Part model, mm, in its own coordinate system. A direction names the side the tool comes from. Coordinates: 2 decimals unless noted, no trailing zeros. Order: outer loops, then holes, each group sorted by start corner. A loop starts at its lowest first (then second) coordinate and runs counter-clockwise, first axis right, second up. Notation, with made-up numbers: M 7,83 L 61,83 A19 cw 61,115 Z; hole C 59.5,-37 d5. An arc over 180 degrees is marked long. Answer in a Markdown table with one row per item. Add a question column.
from build123d import *
from OCP.BRepFilletAPI import BRepFilletAPI_MakeChamfer

# Parameters (mm, degrees)
CROQUIS1_R              = 5.48
CROQUIS1_R_2            = 2.425
SALIENTE_EXTRUIR1_DEPTH = 2.5
CHAFL_N1_SIZE           = 0.4
CHAFL_N1_SIZE2          = 0.692820323
CROQUIS2_R              = 4.265221528
CROQUIS2_R_2            = 3.76303741
SALIENTE_EXTRUIR2_DEPTH = 2.55


with BuildPart() as part:
    # Croquis1 → Saliente-Extruir1 (new, symmetric)
    with BuildSketch(Plane.XY):
        Circle(CROQUIS1_R)
        Circle(CROQUIS1_R_2, mode=Mode.SUBTRACT)
    extrude(amount=SALIENTE_EXTRUIR1_DEPTH, both=True)

    # Chaflán1: one chamfer whose edges measure the first distance from different faces: ONE call of the kernel's chamfer builder (chamfer() names one face for all edges)
    chafl_n1_edges_1 = [part.edges().sort_by_distance(p)[0] for p in [
        (-5.48, 0, -2.5),
    ]]
    chafl_n1_side_1 = [part.faces().sort_by_distance(p)[0] for p in [
        (-5.325002194, 0, -2.5),
    ]]
    chafl_n1_edges_2 = [part.edges().sort_by_distance(p)[0] for p in [
        (-5.48, 0, 2.5),
    ]]
    chafl_n1_side_2 = [part.faces().sort_by_distance(p)[0] for p in [
        (-5.48, 0, 0),
    ]]
    chafl_n1 = BRepFilletAPI_MakeChamfer(part.part.solid().wrapped)
    for e in chafl_n1_edges_1:
        chafl_n1.Add(CHAFL_N1_SIZE, CHAFL_N1_SIZE2, e.wrapped, chafl_n1_side_1[0].wrapped)  # the first distance lies on this face
    for e in chafl_n1_edges_2:
        chafl_n1.Add(CHAFL_N1_SIZE, CHAFL_N1_SIZE2, e.wrapped, chafl_n1_side_2[0].wrapped)  # the first distance lies on this face
    add(Compound.cast(chafl_n1.Shape()), mode=Mode.REPLACE)

    # Croquis2 → Saliente-Extruir2 (add, symmetric)
    with BuildSketch(Plane(origin=(0, 0, 0), x_dir=(-1, 0, 0), z_dir=(0, 0, -1))):
        with Locations(Location((0, 0, 0), (0, 0, 180))):
            Circle(CROQUIS2_R)
        with Locations(Location((0, 0, 0), (0, 0, 180))):
            Circle(CROQUIS2_R_2, mode=Mode.SUBTRACT)
    extrude(amount=SALIENTE_EXTRUIR2_DEPTH, both=True)


solid = part.part
(1) Wall check: line 1 (Y direction, x = 0, z = 0.5) (3 decimals); line 2 (Z direction, x = 1.75, y = -3); line 3 (X direction, y = 0.5, z = -2.2). Give the ranges that are in metal, low to high.
(2) Slice it at C-C (z = 1.1). List the corners of the cut face in (x, y) (3 decimals).
(3) Drop flat-ended pins along their axis: P1, Ø1.5, axis at x = -3, z = 0, coming from the -Y side; P2, Ø3, axis at x = 0, y = 0, coming from the -Z side; P3, Ø6, axis at x = 0, y = 0, coming from the -Z side; P4, Ø3, axis at x = 0, y = -1, coming from the +Z side. Give the stop position or say it passes through.
(4) Pull direction X, two halves, no side cores. Call faces 3 (the flat face through (-4, -2, 2.5)), 4 (the flat face through (0.8, -2.5, -2.5)), 5 (the cylindrical face through (5.227, 1.646, 0.174)): pulls with the +X half, pulls with the -X half, needs draft (parallel to the pull), parting line crosses it, or undercut.
(5) 3-axis set-ups, long thin cutter, end or side, ignore diameter. For faces 1 (the flat face through (0, 4, -2.55)), 2 (the flat face through (0.8, -2.5, 2.5)): which of +Z, -Z, +X, -X, +Y, -Y reach the whole face in a straight line?
(6) Slice it at A-A (x = 0). List the corners of the cut face in (y, z) (3 decimals).
Computed:
| question | item | result |
|---|---|---|
| 1 | line 1 | y = -5.48 to -2.425, 2.425 to 5.48 |
| 1 | line 2 | z = -2.5 to 2.5 |
| 1 | line 3 | x = -5.23 to -2.37, 2.37 to 5.23 |
| 2 | outline | C 0,0 d10.96; hole C 0,0 d4.85 |
| 3 | P1 | stops at y = -5 |
| 3 | P2 | passes through |
| 3 | P3 | stops at z = -2.5 |
| 3 | P4 | stops at z = 2.5 |
| 4 | face 3 | needs draft |
| 4 | face 4 | undercut |
| 4 | face 5 | parting line crosses it |
| 5 | face 1 | -Z, +X, -X, +Y, -Y |
| 5 | face 2 | +Z |
| 6 | outline | M -5.48,-1.807 L -5.08,-2.5 L -4.265,-2.5 L -4.265,-2.55 L -3.763,-2.55 L -3.763,-2.5 L -2.425,-2.5 L -2.425,2.5 L -3.763,2.5 L -3.763,2.55 L -4.265,2.55 L -4.265,2.5 L -4.787,2.5 L -5.48,2.1 Z; M 2.425,-2.5 L 3.763,-2.5 L 3.763,-2.55 L 4.265,-2.55 L 4.265,-2.5 L 5.08,-2.5 L 5.48,-1.807 L 5.48,2.1 L 4.787,2.5 L 4.265,2.5 L 4.265,2.55 L 3.763,2.55 L 3.763,2.5 L 2.425,2.5 Z |
